from build123d import *

# Parameters (mm, degrees)
SKETCH1_R           = 11.5
BOSS_EXTRUDE1_DEPTH = 5


with BuildPart() as part:
    # Sketch1 → Boss-Extrude1 (new body)
    with BuildSketch(Plane.XY):
        with BuildLine():
            Line((58.509519869, -21.974669161), (30.868053734, -14.048606291))
            ThreePointArc((30.868053734, -14.048606291), (20.455340601, -13.329450296), (10.656497706, -16.924510529))
            ThreePointArc((10.656497706, -16.924510529), (0, -20), (-10.656497706, -16.924510529))
            ThreePointArc((-10.656497706, -16.924510529), (-20.455340601, -13.329450296), (-30.868053734, -14.048606291))
            Line((-30.868053734, -14.048606291), (-58.509519869, -21.974669161))
            ThreePointArc((-58.509519869, -21.974669161), (-64.885164476, -18.605521518), (-61.263687445, -12.369745374))
            Line((-61.263687445, -12.369745374), (-36.509479216, -3.359950405))
            ThreePointArc((-36.509479216, -3.359950405), (-17.634305645, 6.764909334), (-2.390807306, 21.81219216))
            ThreePointArc((-2.390807306, 21.81219216), (0, 23), (2.390807306, 21.81219216))
            ThreePointArc((2.390807306, 21.81219216), (17.634305645, 6.764909334), (36.509479216, -3.359950405))
            Line((36.509479216, -3.359950405), (61.263687445, -12.369745374))
            ThreePointArc((61.263687445, -12.369745374), (64.885164476, -18.605521518), (58.509519869, -21.974669161))
        make_face()
        Circle(SKETCH1_R, mode=Mode.SUBTRACT)
    extrude(amount=BOSS_EXTRUDE1_DEPTH)


solid = part.part
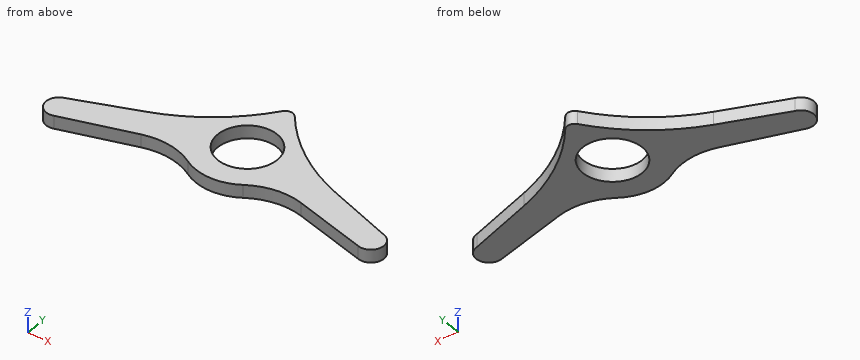
Build history of the part. All positions in model axes, mm. Round coordinates to 2 decimals unless told otherwise and drop trailing zeros. Loops run counter-clockwise (first coordinate to the right, second up) from the corner with the lowest first, then second, coordinate; pieces in that order, holes last. Notation, with made-up numbers: (51.25, 22) -> (76.25, 22) arc R13 ccw to (76.25, 39) -> close; hole circle Ø1 at (86.5, 82). An arc over 180 degrees is marked (long way). Answer in a Markdown table with one row per item.
Item 1: Pin check, flat tips, straight feed: pin 1 (3 mm diameter, centred on x = -5.5, z = 2.5, fed in from -Y); pin 2 (1.5 mm diameter, centred on x = 10.5, z = 4, fed in from +Y). Stop position of each tip, or through.
Answers below:
| item | result |
|---|---|
| pin 1 | stops at y = -19.6 |
| pin 2 | stops at y = 13.47 |
Item 2: Saw through at D-D (y = 15.5). Write the cut outline in (x, z), and give its area (3 significant figures).
Answers below:
| item | result |
|---|---|
| outline | (-7.75, 0) -> (7.75, 0) -> (7.75, 5) -> (-7.75, 5) -> close |
| area | 77.5 mm² |
Item 3: Saw through at A-A (x = 0). Write the cut outline in (y, z), and give its area (3 significant figures).
Answers below:
| item | result |
|---|---|
| outline | (-20, 0) -> (-11.5, 0) -> (-11.5, 5) -> (-20, 5) -> close; (11.5, 0) -> (23, 0) -> (23, 5) -> (11.5, 5) -> close |
| area | 100 mm² |
Item 4: Saw through at C-C (y = -9.5). Write the cut outline in (x, z).
Answers below:
| item | result |
|---|---|
| outline | (-53.38, 0) -> (-6.48, 0) -> (-6.48, 5) -> (-53.38, 5) -> close; (6.48, 0) -> (53.38, 0) -> (53.38, 5) -> (6.48, 5) -> close |
Item 5: Drill centre lines: L1, parallel to Y at x = 0, z = 3.25; L2, parallel to Y at x = 5, z = 3.9; L3, parallel to X at y = 7.5, z = 4.1. Where is each one in solid material? Low to high. Write a range as [from, to].
Answers below:
| item | result |
|---|---|
| L1 | y = [-20, -11.5], [11.5, 23] |
| L2 | y = [-19.36, -10.36], [10.36, 18.56] |
| L3 | x = [-16.65, -8.72], [8.72, 16.65] |
Item 6: Saw through at B-B (z = 2.6). Write the cut outline in (x, y), and give its area (3 significant figures).
Answers below:
| item | result |
|---|---|
| outline | (-61.26, -12.37) arc R5 ccw (long way) to (-58.51, -21.97) -> (-30.87, -14.05) arc R25 cw to (-10.66, -16.92) arc R20 ccw to (10.66, -16.92) arc R25 cw to (30.87, -14.05) -> (58.51, -21.97) arc R5 ccw (long way) to (61.26, -12.37) -> (36.51, -3.36) arc R75 cw to (2.39, 21.81) arc R3 ccw to (-2.39, 21.81) arc R75 cw to (-36.51, -3.36) -> close; hole circle Ø23 at (0, 0) |
| area | 1,900 mm² |
